Read the model definition and answer for the solid it produces. Units are mm, in the model's axes. Face numbers are marked on the shaded views. A direction names the side the tool comes from. Round coordinates to 2 decimals unless told otherwise and drop trailing zeros. Order: outer loops, then holes, each group sorted by start corner. A loop starts at its lowest first (then second) coordinate and runs counter-clockwise, first axis right, second up. Notation, with made-up numbers: (-35.5, 63.25) -> (6.5, 63.25) arc R30 cw to (6.5, 89.25) -> close; hole circle Ø1 at (88, -31). An arc over 180 degrees is marked (long way). One line per item, written item: value. Start each with the question number.
1. Section A-A (x = -2.5) is taken. Give the vertices of the cut face in (y, z).
2. For the marked faces 1, 2, 3, 4 and 5, determine the directions among +Z, -Z, +X, -X, +Y, -Y from which every point of the face is accessible in a straight line to the end or side of a thin tool.
3. Consider line 1 (Z direction, x = 9.5, y = -7.5); line 2 (Y direction, x = 3, z = 20.5). Determine where each line is inside the solid, lowest interval first.
4. Section C-C (z = 11.5) is taken. Give the vertices of the cut face in (x, y), then the cut area to 3 significant figures.
5. Flat-ended cylindrical pins translate along their axes: pin 1 Ø4 at (x, z) = (15, 0) entering from -Y; pin 2 Ø3 at (x, z) = (4, 19) entering from -Y; pin 3 Ø6 at (y, z) = (-2, 19) entering from +X. Find the tip coordinate at first contact, or state that the pin passes through.
6. Section B-B (y = -1.25) is taken. Give the vertices of the cut face in (x, z).
7. Section D-D (x = 11) is taken. Give the vertices of the cut face in (y, z), then the cut area to 3 significant figures.
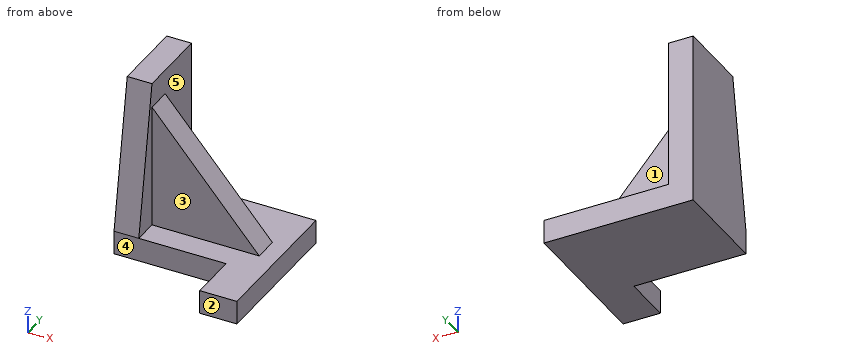
from build123d import *

# Parameters (mm, degrees)
F1_DEPTH = 5
F3_DEPTH = 5
F4_W     = 7.5
F4_H     = 10
F5_DEPTH = 4.8


with BuildPart() as f1:
    # F0 (on Front) → F1 (new body)
    with BuildSketch(Plane.XZ):
        Polygon((21.644296, 0), (0, 25), (0, 0), align=None)
    extrude(amount=F1_DEPTH)

    # F2 (on Right) → F3 (join)
    with BuildSketch(Plane.YZ):
        Polygon((-10, 0), (10, 0), (10, 30), (-5, 30), align=None)
    extrude(amount=-F3_DEPTH)

    # F4 (on Top) → F5 (join)
    with BuildSketch(Plane.XY):
        Polygon((-5, 10), (-5, -10), (17.615132, -10), (25.115132, -10), (25.115132, 10), align=None)
        with Locations((21.365132, -15)):
            Rectangle(F4_W, F4_H)
    extrude(amount=-F5_DEPTH)


solid = f1.part
Answer:
1. outline: (-10, -4.8) -> (10, -4.8) -> (10, 30) -> (-5, 30) -> (-10, 0) -> close
2. face 1: +Z, +X, +Y
2. face 2: +Z, -Z, +X, -X, -Y
2. face 3: +Z, +X, -Y
2. face 4: +Z, -Z, -X, -Y
2. face 5: +Z, +X
3. line 1: -4.8 to 0
3. line 2: -5 to 0
4. outline: (-5, -8.08) -> (0, -8.08) -> (0, -5) -> (11.69, -5) -> (11.69, 0) -> (0, 0) -> (0, 10) -> (-5, 10) -> close
4. area: 149 mm^2
5. pin 1: y = -10
5. pin 2: y = -5
5. pin 3: x = 7.79
6. outline: (-5, -4.8) -> (25.12, -4.8) -> (25.12, 0) -> (21.64, 0) -> (0, 25) -> (0, 30) -> (-5, 30) -> close
7. outline: (-10, -4.8) -> (10, -4.8) -> (10, 0) -> (0, 0) -> (0, 12.29) -> (-5, 12.29) -> (-5, 0) -> (-10, 0) -> close
7. area: 157 mm^2
